Study the drawing (mm; zero at the part's minimum x, y, z) and answer. A direction names the side the tool comes from. Round coordinates to 2 decimals unless told otherwise and drop trailing zeros. Write each loop counter-clockwise with the first axis right and the second up, starting at its lowest first coordinate (ties: lowest second). Pieces come first, ordered by that corner, then holes.
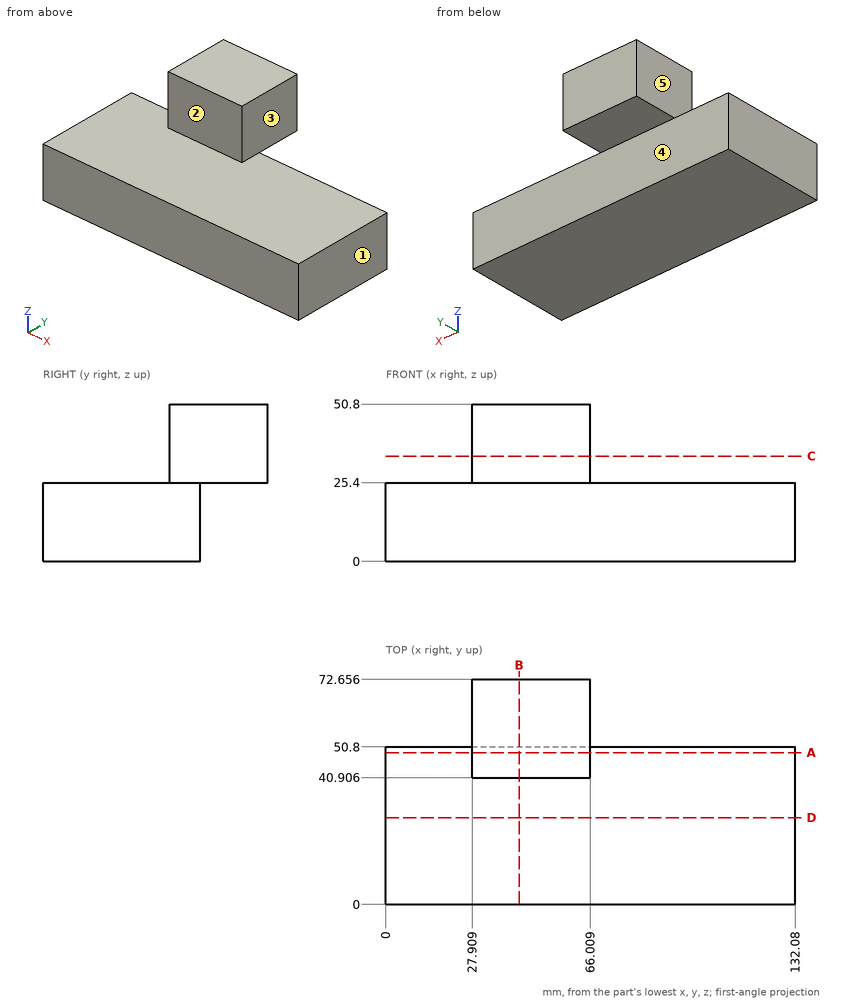
1. A tool of negligible diameter and unlimited length cuts with its end or side. For the marked faces 1, 2, 3, 4 and 5, from which of +Z, -Z, +X, -X, +Y, -Y can it reach the whole face along a straight path? Write none if from no direction.
Geometry says:
face 1: +Z, -Z, +X, +Y, -Y
face 2: +Z, +X, -X, -Y
face 3: +Z, +X, +Y, -Y
face 4: -Z, +X, -X, +Y
face 5: +Z, -X, +Y, -Y
2. Straight lines are drawn through the part: line 1 along X through (y, z) = (47.5, 39); line 2 along Y through (x, z) = (116.5, 12.5); line 3 along Z through (x, y) = (107.5, 17.5). For each, find the intervals that lie inside material, in ascending order.
Geometry says:
line 1: x = 27.91 to 66.01
line 2: y = 0 to 50.8
line 3: z = 0 to 25.4
3. Section C-C on z = 34 is taken. Determine the outline of the cut face in (x, y).
Geometry says:
outline: (27.91, 40.91) - (66.01, 40.91) - (66.01, 72.66) - (27.91, 72.66) - close
4. Section A-A on y = 49 is taken. Determine the outline of the cut face in (x, z), plus the area to 3 significant figures.
Geometry says:
outline: (0, 0) - (132.08, 0) - (132.08, 25.4) - (66.01, 25.4) - (66.01, 50.8) - (27.91, 50.8) - (27.91, 25.4) - (0, 25.4) - close
area: 4,320 mm2
5. Given pin 1 (6.5 mm diameter, centred on x = 44.5, y = 66.5, fed in from -Z); pin 2 (2 mm diameter, centred on y = 39.5, z = 32.5, fed in from +X); pin 3 (7.5 mm diameter, centred on y = 52, z = 34, fed in from -X); pin 4 (7.5 mm diameter, centred on x = 75.5, z = 16, fed in from +Y), each flat-ended and moving along its own axis, determine where each tip first touches the part or whether it passes through.
Geometry says:
pin 1: stops at z = 25.4
pin 2: passes through
pin 3: stops at x = 27.91
pin 4: stops at y = 50.8
6. Section D-D on y = 28 is taken. Determine the outline of the cut face in (x, z).
Geometry says:
outline: (0, 0) - (132.08, 0) - (132.08, 25.4) - (0, 25.4) - close
7. Section B-B on x = 43 is taken. Determine the outline of the cut face in (y, z), plus the area to 3 significant figures.
Geometry says:
outline: (0, 0) - (50.8, 0) - (50.8, 25.4) - (72.66, 25.4) - (72.66, 50.8) - (40.91, 50.8) - (40.91, 25.4) - (0, 25.4) - close
area: 2,100 mm2
